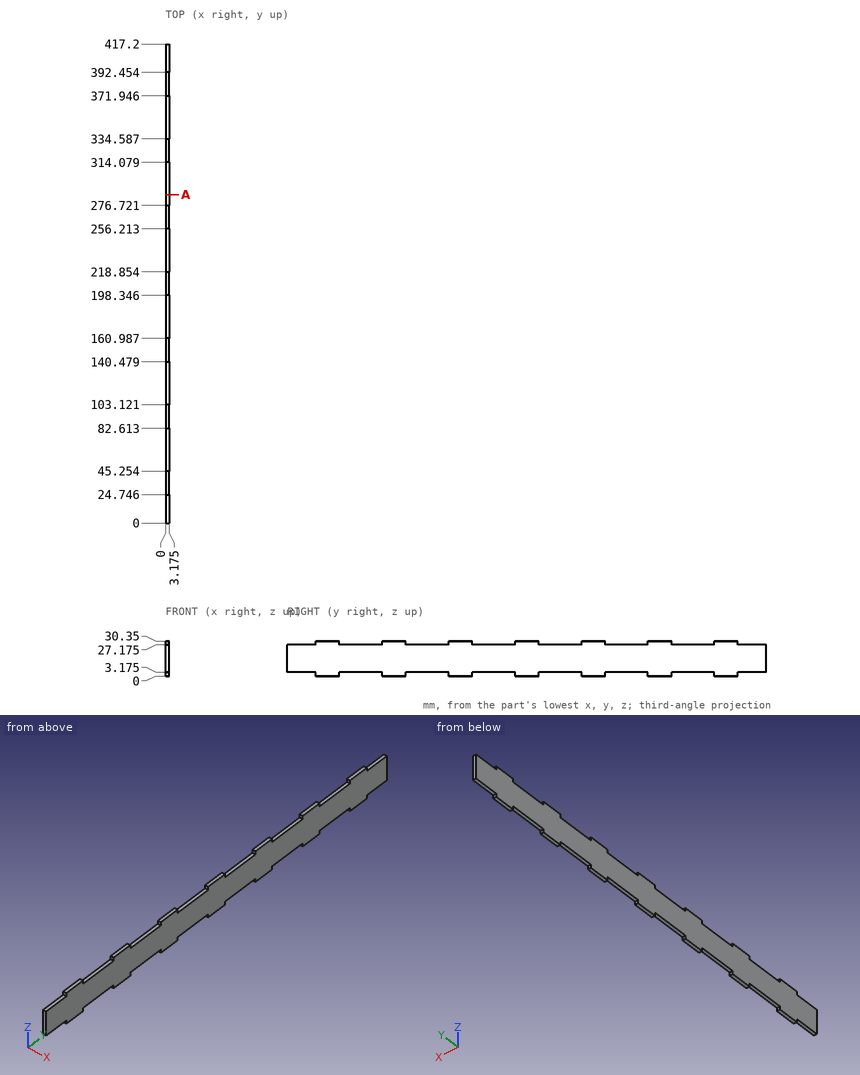
Job drawing, mm, ordinate dimensions from the low corner. One solid piece. Round coordinates to 2 decimals unless told otherwise and drop trailing zeros. Loops run counter-clockwise (first coordinate to the right, second up) from the corner with the lowest first, then second, coordinate; pieces in that order, holes last. Notation, with made-up numbers: M 83,11.25 L 136,11.25 A13 cw 136,23.25 Z; hole C 68,-1.75 d2. An arc over 180 degrees is marked long. One line per question, with ' | ' between items. Start each with the question number.
Item 1: Cut at A-A, the plane y = 286. Write the cut outline in (x, z) (1 decimal), plus the area to 3 significant figures.
Item 2: Wall check: line 1 (Z direction, x = 1.5, y = 171.5) (1 decimal). Give the ranges that are in metal, low to high.
Item 3: Pin check, flat tips, straight feed: pin 1 Ø1.6 at (x, z) = (1.5, 2) entering from +Y; pin 2 Ø1 at (x, z) = (1.5, 2.5) entering from -Y; pin 3 Ø1 at (x, y) = (2.5, 123.5) entering from -Z (3 decimals). Stop position of each tip, or through.
Responses:
1) outline: M 0,3.2 L 3.2,3.2 L 3.2,27.2 L 0,27.2 Z | area: 76.2 mm²
2) line 1: z = 3.2 to 27.2
3) pin 1: stops at y = 392.45 | pin 2: stops at y = 24.75 | pin 3: stops at z = 3.175
